from build123d import *

# Parameters (mm, degrees)
SKETCH1_W                    = 30
SKETCH1_H                    = 15
BASE_FLANGE1_DEPTH           = 3.175
EDGE_FLANGE1_STRIP_W         = 18.7
EDGE_FLANGE1_STRIP_H         = 3.175
EDGE_FLANGE1_STRIP_CUT_DEPTH = 15
EDGE_FLANGE1_DEPTH           = 15
EDGE_FLANGE2_STRIP_W         = 18.7
EDGE_FLANGE2_STRIP_H         = 3.175
EDGE_FLANGE2_STRIP_CUT_DEPTH = 15
EDGE_FLANGE2_DEPTH           = 15
SKETCH14_R                   = 5.08
CUT_EXTRUDE1_DEPTH           = 82.072299394
SKETCH15_R                   = 2.54
CUT_EXTRUDE2_DEPTH           = 10
FILLET1_R                    = 3


# Sheet-metal steps are written as plain solids
with BuildPart() as part:
    # Sketch1 → Base-Flange1 (new body)
    with BuildSketch(Plane.XY):
        Rectangle(SKETCH1_W, SKETCH1_H)
    extrude(amount=-BASE_FLANGE1_DEPTH)

    # Edge-Flange1 strip (across the edge) → Edge-Flange1 strip cut (cut)
    with BuildSketch(Plane(origin=(15, -7.5, 0), x_dir=(-1, 0, 0), z_dir=(0, 1, 0))):
        with Locations((-6.35, -1.5875)):
            Rectangle(EDGE_FLANGE1_STRIP_W, EDGE_FLANGE1_STRIP_H)
    extrude(amount=EDGE_FLANGE1_STRIP_CUT_DEPTH, mode=Mode.SUBTRACT)

    # Edge-Flange1 section (across the edge) → Edge-Flange1 (add)
    with BuildSketch(Plane(origin=(15, -7.5, 0), x_dir=(-1, 0, 0), z_dir=(0, 1, 0))):
        with BuildLine():
            Line((-3.175, 3), (-3.175, 75.477))
            Line((-3.175, 75.477), (0, 75.477))
            Line((0, 75.477), (0, 3))
            ThreePointArc((0, 3), (0.878679656, 0.878679656), (3, 0))
            Line((3, 0), (3, -3.175))
            ThreePointArc((3, -3.175), (-1.366384374, -1.366384374), (-3.175, 3))
        make_face()
    extrude(amount=EDGE_FLANGE1_DEPTH)

    # Edge-Flange2 strip (across the edge) → Edge-Flange2 strip cut (cut)
    with BuildSketch(Plane(origin=(15, -7.5, 75.477), x_dir=(0, 0, -1), z_dir=(0, 1, 0))):
        with Locations((-6.35, -1.5875)):
            Rectangle(EDGE_FLANGE2_STRIP_W, EDGE_FLANGE2_STRIP_H)
    extrude(amount=EDGE_FLANGE2_STRIP_CUT_DEPTH, mode=Mode.SUBTRACT)

    # Edge-Flange2 section (across the edge) → Edge-Flange2 (add)
    with BuildSketch(Plane(origin=(15, -7.5, 75.477), x_dir=(0, 0, -1), z_dir=(0, 1, 0))):
        with BuildLine():
            Line((-3.175, 3), (-3.175, 26.825))
            Line((-3.175, 26.825), (0, 26.825))
            Line((0, 26.825), (0, 3))
            ThreePointArc((0, 3), (0.878679656, 0.878679656), (3, 0))
            Line((3, 0), (3, -3.175))
            ThreePointArc((3, -3.175), (-1.366384374, -1.366384374), (-3.175, 3))
        make_face()
    extrude(amount=EDGE_FLANGE2_DEPTH)

    # Sketch14 → Cut-Extrude1 (cut, through all)
    with BuildSketch(Plane.XY):
        with Locations((-7.38, 0)):
            Circle(SKETCH14_R)
    extrude(amount=-CUT_EXTRUDE1_DEPTH, mode=Mode.SUBTRACT)

    # Sketch15 → Cut-Extrude2 (cut)
    with BuildSketch(Plane.XY.offset(78.652)):
        with Locations((-6.745, 0)):
            Circle(SKETCH15_R)
    extrude(amount=-CUT_EXTRUDE2_DEPTH, mode=Mode.SUBTRACT)

    # Fillet1
    fillet1_edges = [part.edges().sort_by_distance(p)[0] for p in [
        (-11.825, -7.5, 77.0645),
        (-11.825, 7.5, 77.0645),
        (-15, -7.5, -1.5875),
        (-15, 7.5, -1.5875),
    ]]
    fillet(fillet1_edges, radius=FILLET1_R)


solid = part.part
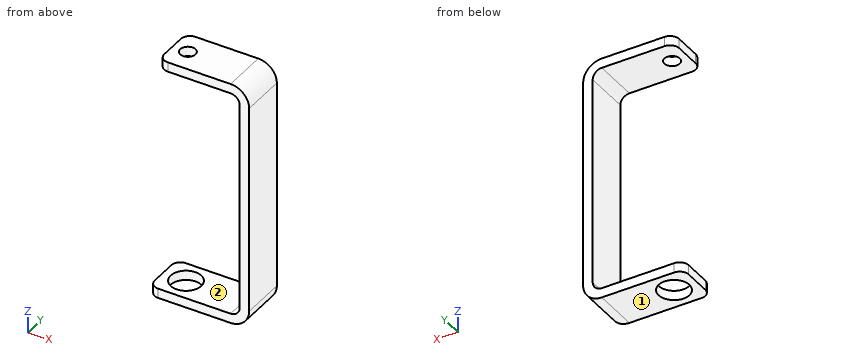
Check sheet for the modelled part. Datum: model origin and axes. Units: mm. Face numbers are marked on the shaded views. A direction names the side the tool comes from. Coordinates: 2 decimals unless noted, no trailing zeros. Loops run counter-clockwise (first coordinate to the right, second up) from the corner with the lowest first, then second, coordinate; pieces in that order, holes last. Notation, with made-up numbers: (24, 34.25) -> (55, 34.25) arc R28 ccw to (55, 66.25) -> close; hole circle Ø7 at (86.5, 88.5). An arc over 180 degrees is marked (long way). Answer in a Markdown table with one row per item.
1. Access from +Z, -Z, +X, -X, +Y, -Y to the whole of each face (thin tool, end or side, straight path). Record for the marked faces 1 and 2.
Check values:
| item | result |
|---|---|
| face 1 | -Z, +X, -X, +Y, -Y |
| face 2 | -X, +Y, -Y |
2. Sectioned sample at C-C, the plane x = -7.38. Record the boundary of the cut face in (y, z) (3 decimals).
Check values:
| item | result |
|---|---|
| outline | (-7.5, -3.175) -> (-5.08, -3.175) -> (-5.08, 0) -> (-7.5, 0) -> close; (-7.5, 75.477) -> (-2.459, 75.477) -> (-2.459, 78.652) -> (-7.5, 78.652) -> close; (2.459, 75.477) -> (7.5, 75.477) -> (7.5, 78.652) -> (2.459, 78.652) -> close; (5.08, -3.175) -> (7.5, -3.175) -> (7.5, 0) -> (5.08, 0) -> close |
3. Go/stop test with flat-tipped pins: pin 1 (5 mm diameter, centred on y = 0, z = 44, fed in from -X); pin 2 (1.6 mm diameter, centred on y = -1.5, z = 77.5, fed in from -X) (3 decimals); pin 3 (10 mm diameter, centred on x = 6, z = 12.5, fed in from -Y). Record where each tip stops, or that it passes through.
Check values:
| item | result |
|---|---|
| pin 1 | stops at x = 15 |
| pin 2 | stops at x = -11.825 |
| pin 3 | passes through |
4. Sectioned sample at B-B, the plane x = 3. Record the boundary of the cut face in (y, z) (3 decimals), then the cut area to 4 significant figures.
Check values:
| item | result |
|---|---|
| outline | (-7.5, -3.175) -> (7.5, -3.175) -> (7.5, 0) -> (-7.5, 0) -> close; (-7.5, 75.477) -> (7.5, 75.477) -> (7.5, 78.652) -> (-7.5, 78.652) -> close |
| area | 95.25 mm2 |
5. Sectioned sample at A-A, the plane y = 0. Record the boundary of the cut face in (x, z) (3 decimals).
Check values:
| item | result |
|---|---|
| outline | (-15, -3.175) -> (-12.46, -3.175) -> (-12.46, 0) -> (-15, 0) -> close; (-11.825, 75.477) -> (-9.285, 75.477) -> (-9.285, 78.652) -> (-11.825, 78.652) -> close; (-4.205, 75.477) -> (12, 75.477) arc R3 cw to (15, 72.477) -> (15, 3) arc R3 cw to (12, 0) -> (-2.3, 0) -> (-2.3, -3.175) -> (12, -3.175) arc R6.175 ccw to (18.175, 3) -> (18.175, 72.477) arc R6.175 ccw to (12, 78.652) -> (-4.205, 78.652) -> close |
6. Material ranges on line 1 along Z through (x, y) = (7, -4.75) (3 decimals); line 2 along Y through (x, z) = (-7.38, -1.65); line 3 along X through (y, z) = (0, 3) (3 decimals), recorded low to high. Write a range as [from, to].
Check values:
| item | result |
|---|---|
| line 1 | z = [-3.175, 0], [75.477, 78.652] |
| line 2 | y = [-7.5, -5.08], [5.08, 7.5] |
| line 3 | x = [15, 18.175] |
7. Sectioned sample at D-D, the plane z = 22. Record the boundary of the cut face in (x, y) (3 decimals).
Check values:
| item | result |
|---|---|
| outline | (15, -7.5) -> (18.175, -7.5) -> (18.175, 7.5) -> (15, 7.5) -> close |
